Study the drawing (mm; zero at the part's minimum x, y, z) and answer. A direction names the side the tool comes from. Coordinates: 2 decimals unless noted, no trailing zeros. Order: outer loops, then holes, each group sorted by start corner. A loop starts at its lowest first (then second) coordinate and runs counter-clockwise, first axis right, second up. Notation, with made-up numbers: M 58.25,26.5 L 78.25,26.5 A20 ccw 78.25,37.5 Z; hole C 88.25,57 d7. An arc over 180 degrees is marked long. One line per item, written item: value. Start each with the question number.
Q1. The part is cut by section A-A on z = 7.5. Give the vertices of the cut face in (x, y), then the cut area to 3 significant figures.
Q2. The part is cut by section D-D on x = 22. Give the vertices of the cut face in (y, z) (1 decimal).
Q3. The part is cut by section C-C on z = 10.25. Give the vertices of the cut face in (x, y).
Q4. Straight lines are drawn through the part: line 1 along X through (y, z) = (15.5, 4); line 2 along Z through (x, y) = (5.25, 14.5); line 3 along X through (y, z) = (6, 15.25) (1 decimal). For each, find the intervals that lie inside material, in ascending order. Write a range as [from, to].
Q5. Determine the mould class of the marked faces 4, 5 and 6 for opening direction X: pulls with the +X half, pulls with the -X half, needs draft (parallel to the pull), parting line crosses it, or undercut.
Q6. For the marked faces 1, 2 and 3, determine the directions among +Z, -Z, +X, -X, +Y, -Y from which every point of the face is accessible in a straight line to the end or side of a thin tool.
Q7. Each of these flat-tipped pins is pushed along its axis until it touches: pin 1 Ø1 at (x, z) = (15.5, 11) entering from +Y (1 decimal); pin 2 Ø5 at (x, y) = (7.5, 12.5) entering from -Z. Where does it stop, or does it pass through?
Q8. The part is cut by section B-B on y = 18. Give the vertices of the cut face in (x, z), then the cut area to 3 significant figures.
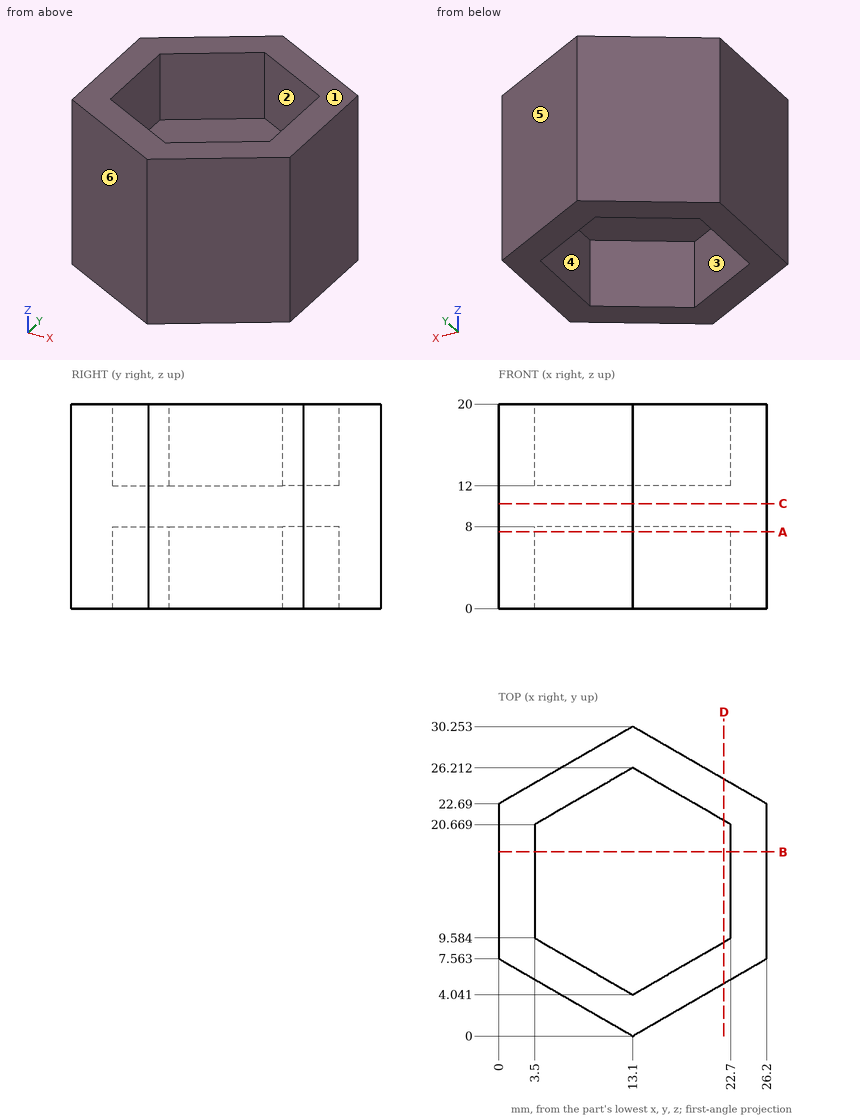
Output:
1. outline: M 0,7.56 L 13.1,0 L 26.2,7.56 L 26.2,22.69 L 13.1,30.25 L 0,22.69 Z; hole M 3.5,9.58 L 13.1,4.04 L 22.7,9.58 L 22.7,20.67 L 13.1,26.21 L 3.5,20.67 Z
1. area: 275 mm^2
2. outline: M 5.1,0 L 9.2,0 L 9.2,8 L 21.1,8 L 21.1,0 L 25.1,0 L 25.1,20 L 21.1,20 L 21.1,12 L 9.2,12 L 9.2,20 L 5.1,20 Z
3. outline: M 0,7.56 L 13.1,0 L 26.2,7.56 L 26.2,22.69 L 13.1,30.25 L 0,22.69 Z
4. line 1: x = [0, 3.5], [22.7, 26.2]
4. line 2: z = [8, 12]
4. line 3: x = [2.7, 9.7], [16.5, 23.5]
5. face 4: undercut
5. face 5: pulls with the +X half
5. face 6: pulls with the -X half
6. face 1: +Z, +X, -X, +Y, -Y
6. face 2: +Z
6. face 3: -Z
7. pin 1: stops at y = 29.2
7. pin 2: stops at z = 8
8. outline: M 0,0 L 3.5,0 L 3.5,8 L 22.7,8 L 22.7,0 L 26.2,0 L 26.2,20 L 22.7,20 L 22.7,12 L 3.5,12 L 3.5,20 L 0,20 Z
8. area: 217 mm^2
